Can you work these out from the drawing? Everything is in mm from the part's minimum corner. Coordinates: 2 decimals unless noted, no trailing zeros. Loops run counter-clockwise (first coordinate to the right, second up) from the corner with the lowest first, then second, coordinate; pieces in that order, holes last. Notation, with made-up numbers: (78, -16.5) -> (109, -16.5) arc R32 ccw to (109, 19.5) -> close; hole circle Ø1 at (13.25, -3.5). An arc over 180 degrees is marked (long way). One line per question, with ' | ' between items.
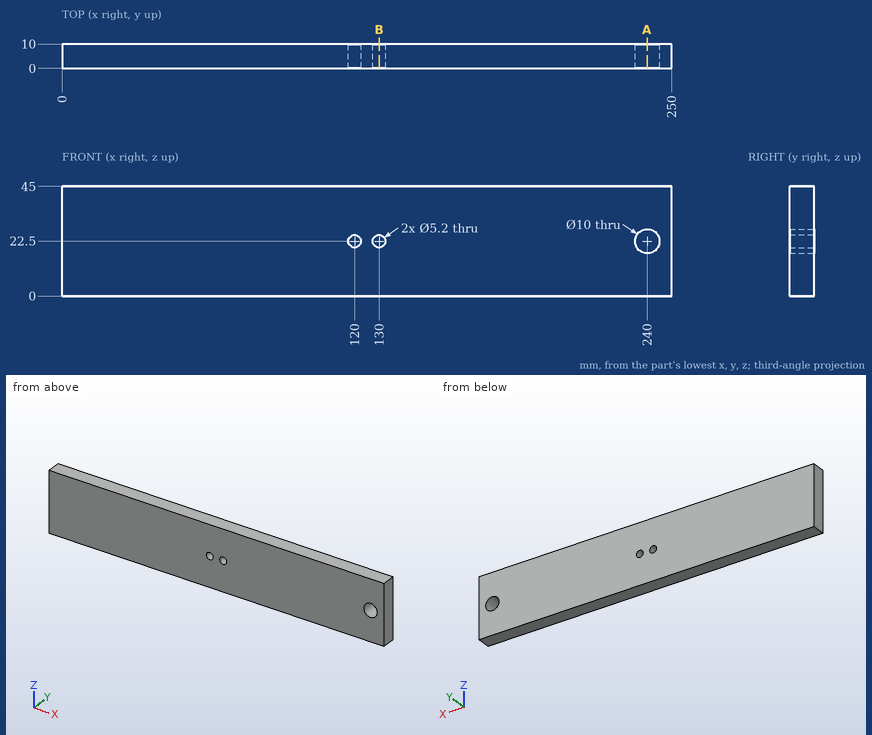
Q1. For pin 1 (12 mm diameter, centred on x = 145.5, z = 32.5, fed in from -Y), with a flat end and sliding along its axis, tell me the tip position at first contact or that it passes through.
Values follow:
pin 1: stops at y = 0
Q2. Imagine slicing it at A-A on x = 240. Write out the boundary of the cut face in (y, z), plus the area to 3 significant figures.
Values follow:
outline: (0, 0) -> (10, 0) -> (10, 17.5) -> (0, 17.5) -> close; (0, 27.5) -> (10, 27.5) -> (10, 45) -> (0, 45) -> close | area: 350 mm2
Q3. Imagine slicing it at B-B on x = 130. Write out the boundary of the cut face in (y, z), plus the area to 3 significant figures.
Values follow:
outline: (0, 0) -> (10, 0) -> (10, 19.9) -> (0, 19.9) -> close; (0, 25.1) -> (10, 25.1) -> (10, 45) -> (0, 45) -> close | area: 398 mm2
Q4. Please list where these lines run through material, in increasing order: L1, parallel to X at y = 3, z = 22.5; L2, parallel to Z at x = 240, y = 4; L3, parallel to Z at x = 130.5, y = 8. Write a range as [from, to].
Values follow:
L1: x = [0, 117.4], [122.6, 127.4], [132.6, 235], [245, 250] | L2: z = [0, 17.5], [27.5, 45] | L3: z = [0, 19.95], [25.05, 45]
